from build123d import *

# Parameters (mm, degrees)
SKETCH1_R           = 1.778
SKETCH1_W           = 25.4
SKETCH1_H           = 5.842
BOSS_EXTRUDE1_DEPTH = 5.842
SKETCH2_W           = 63.5
SKETCH2_H           = 6.757924
BOSS_EXTRUDE2_DEPTH = 5.842
FILLET1_R           = 3.175
SKETCH4_R           = 3.175
SKETCH4_W           = 2.975
SKETCH4_H           = 6.35
CUT_EXTRUDE2_DEPTH  = 95.65387769
CUT_EXTRUDE3_DEPTH  = 95.65387769
BOSS_EXTRUDE4_START = -5.842
SKETCH7_R           = 2.0828
BOSS_EXTRUDE4_DEPTH = 5.842
FILLET12_R          = 12.7
SKETCH8_R           = 2.0828
BOSS_EXTRUDE5_DEPTH = 5.842
FILLET13_R          = 3.175
SKETCH9_R           = 2.0828
CUT_EXTRUDE4_DEPTH  = 107.047047485


with BuildPart() as part:
    # Sketch1 → Boss-Extrude1 (new body)
    with BuildSketch(Plane.XY):
        Polygon((0, 12.7), (-5.842, 12.7), (-5.842, 0), (0, 0), (0, -12.7), (-5.842, -12.7), (-5.842, -25.4), (0, -25.4), (0, -25.908), (12.7, -25.908), (12.7, -31.75), (0, -31.75), (0, -38.1), (-5.842, -38.1), (-5.842, -50.8), (0, -50.8), (0, -57.349898), (12.7, -57.349898), (12.7, -63.191898), (25.4, -63.191898), (25.4, -57.349898), (50.8, -57.349898), (50.8, -63.191898), (63.5, -63.191898), (63.5, 17.55013), (0, 17.55013), align=None)
        with Locations((19.065986419, -60.397898)):
            Circle(SKETCH1_R, mode=Mode.SUBTRACT)
        with Locations((19.05, -28.702)):
            Circle(SKETCH1_R, mode=Mode.SUBTRACT)
        with Locations((57.157993209, -60.397898)):
            Circle(SKETCH1_R, mode=Mode.SUBTRACT)
        with Locations((38.1, -28.829)):
            Rectangle(SKETCH1_W, SKETCH1_H, mode=Mode.SUBTRACT)
        with Locations((57.15, -28.702)):
            Circle(SKETCH1_R, mode=Mode.SUBTRACT)
    extrude(amount=BOSS_EXTRUDE1_DEPTH)

    # Sketch2 → Boss-Extrude2 (add)
    with BuildSketch(Plane.XY.offset(5.842)):
        with Locations((31.75, -66.57086)):
            Rectangle(SKETCH2_W, SKETCH2_H)
    extrude(amount=-BOSS_EXTRUDE2_DEPTH)

    # Fillet1
    fillet1_edges = [part.edges().sort_by_distance(p)[0] for p in [
        (63.5, -69.949822, 2.921),
    ]]
    fillet(fillet1_edges, radius=FILLET1_R)

    # Sketch4 → Cut-Extrude2 (cut, through all)
    with BuildSketch(Plane.XY.offset(5.842)):
        with Locations((38.1, 9.61263)):
            Circle(SKETCH4_R)
        with Locations((23.9125, -6.35)):
            Rectangle(SKETCH4_W, SKETCH4_H)
        with Locations((23.9125, -19.05)):
            Rectangle(SKETCH4_W, SKETCH4_H)
        with Locations((52.2875, -19.05)):
            Rectangle(SKETCH4_W, SKETCH4_H)
        with Locations((52.2875, -6.35)):
            Rectangle(SKETCH4_W, SKETCH4_H)
    extrude(amount=-CUT_EXTRUDE2_DEPTH, mode=Mode.SUBTRACT)

    # Sketch5 → Cut-Extrude3 (cut, through all)
    with BuildSketch(Plane.XY.offset(5.842)):
        with BuildLine():
            Line((7.9375, 8.02513), (17.4625, 8.02513))
            ThreePointArc((17.4625, 8.02513), (20.6375, 4.85013), (17.4625, 1.67513))
            Line((17.4625, 1.67513), (7.9375, 1.67513))
            ThreePointArc((7.9375, 1.67513), (4.7625, 4.85013), (7.9375, 8.02513))
        make_face()
        with BuildLine():
            Line((7.9375, -1.62687), (17.4625, -1.62687))
            ThreePointArc((17.4625, -1.62687), (20.6375, -4.80187), (17.4625, -7.97687))
            Line((17.4625, -7.97687), (7.9375, -7.97687))
            ThreePointArc((7.9375, -7.97687), (4.7625, -4.80187), (7.9375, -1.62687))
        make_face()
        with BuildLine():
            Line((7.9375, -11.27887), (17.4625, -11.27887))
            ThreePointArc((17.4625, -11.27887), (20.6375, -14.45387), (17.4625, -17.62887))
            Line((17.4625, -17.62887), (7.9375, -17.62887))
            ThreePointArc((7.9375, -17.62887), (4.7625, -14.45387), (7.9375, -11.27887))
        make_face()
    extrude(amount=-CUT_EXTRUDE3_DEPTH, mode=Mode.SUBTRACT)

    # Sketch7 → Boss-Extrude4 (add)
    with BuildSketch(Plane.XY.offset(5.842).offset(BOSS_EXTRUDE4_START)):
        with BuildLine():
            Line((60.544173966, -77.950003252), (55.218486469, -69.949822))
            Line((55.218486469, -69.949822), (60.325, -69.949822))
            ThreePointArc((60.325, -69.949822), (62.57006403, -69.01988603), (63.5, -66.774822))
            Line((63.5, -66.774822), (67.615323654, -70.182525218))
            ThreePointArc((67.615323654, -70.182525218), (68.150012892, -77.771642798), (60.544173966, -77.950003252))
        make_face()
        with Locations((64.262, -74.232177218)):
            Circle(SKETCH7_R, mode=Mode.SUBTRACT)
    extrude(amount=BOSS_EXTRUDE4_DEPTH)

    # Fillet12
    fillet12_edges = [part.edges().sort_by_distance(p)[0] for p in [
        (55.218486469, -69.949822, 2.921),
        (63.5, -66.774822, 2.921),
    ]]
    fillet(fillet12_edges, radius=FILLET12_R)

    # Sketch8 → Boss-Extrude5 (add)
    with BuildSketch(Plane.XY.offset(5.842)):
        with BuildLine():
            Line((64.693546, -17.610328), (63.5, -17.610328))
            Line((63.5, -17.610328), (63.5, -17.473065939))
            ThreePointArc((63.5, -17.473065939), (59.435746, -12.352528), (63.5, -7.231990061))
            Line((63.5, -7.231990061), (63.5, -7.094728))
            Line((63.5, -7.094728), (64.693546, -7.094728))
            ThreePointArc((64.693546, -7.094728), (69.951346, -12.352528), (64.693546, -17.610328))
        make_face()
        with Locations((64.693546, -12.352528)):
            Circle(SKETCH8_R, mode=Mode.SUBTRACT)
    extrude(amount=-BOSS_EXTRUDE5_DEPTH)

    # Fillet13
    # the kernel refuses this fillet: 3.175 mm, written as the material it adds along each edge
    with BuildSketch(Plane(origin=(63.5, -7.094728, 5.842), x_dir=(0, 1, 0), z_dir=(0, 0, -1))) as fillet13_piece_1:
        with BuildLine():
            CenterArc((2.938903965, 3.175), FILLET13_R, 193.589847282, 76.410152718)
            Line((-0.147204456, 2.428970633), (-0.455815298, 2.354367696))
            ThreePointArc((-0.455815298, 2.354367696), (-0.3175, 1.193546), (-0.3175, 0))
            Line((-0.3175, 0), (0, -0.3175))
            Line((0, -0.3175), (2.938903965, -0.3175))
            Line((2.938903965, -0.3175), (2.938903965, 0))
        make_face()
    extrude(amount=5.842)
    with BuildSketch(Plane(origin=(63.5, -17.610328, 5.842), x_dir=(0.9981686426778995, 0.0604926505830248, 0), z_dir=(0, 0, -1))) as fillet13_piece_2:
        with BuildLine():
            CenterArc((2.99140335, 3.125585947), FILLET13_R, 183.468090933, 76.410152718)
            Line((-0.177782091, 2.933521781), (-0.494700635, 2.914315365))
            Line((-0.494700635, 2.914315365), (-0.316918544, -0.019206417))
            Line((-0.316918544, -0.019206417), (0.019206417, -0.316918544))
            ThreePointArc((0.019206417, -0.316918544), (1.210566607, -0.244717783), (2.377629483, -0.312558595))
            Line((2.377629483, -0.312558595), (2.433427107, 0))
        make_face()
    extrude(amount=5.842)
    # the kernel refuses this fillet: 3.175 mm, written as the material it takes off along each edge

    # Sketch9 → Cut-Extrude4 (cut, through all)
    with BuildSketch(Plane.XY.offset(5.842)):
        with Locations((64.693546, -12.352528)):
            Circle(SKETCH9_R)
    extrude(amount=-CUT_EXTRUDE4_DEPTH, mode=Mode.SUBTRACT)


solid = part.part
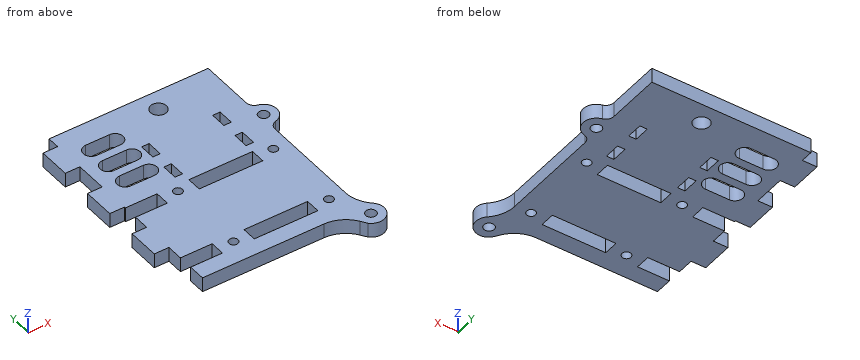
Geometry: final body of the model. Coordinates: model frame, mm. Round coordinates to 2 decimals unless told otherwise and drop trailing zeros. Loops run counter-clockwise (first coordinate to the right, second up) from the corner with the lowest first, then second, coordinate; pieces in that order, holes last.
Q1. Material intervals for L1, parallel to Y at x = 2.5, z = 4.9; L2, parallel to Y at x = 22.5, z = 0.3 (3 decimals); L3, parallel to Y at x = 20, z = 3.55, sorted ascending.
Q2. Section D-D on y = -46. Return loops of the section in (x, z), plus the area to 3 significant figures.
Q3. Section A-A on x = 32.5. Return loops of the section in (y, z).
Q4. Pin query (flat end, axial travel): P1, Ø1, axis at x = 36, z = 1.5, coming from the -Y side; P2, Ø2.5, axis at x = 52, z = 4, coming from the -Y side; P3, Ø1.8, axis at x = -2, z = 2, coming from the +Y side. Return the tip coordinate at first contact, or that it passes through.
Q5. Section B-B on x = 19.05. Return loops of the section in (y, z).
Q6. Section C-C on x = 57.15. Return loops of the section in (y, z).
Evaluation:
1. L1: y = -69.95 to -63.19, -57.35 to -31.75, -25.91 to 17.55
1. L2: y = -69.95 to -22.225, -15.875 to -9.525, -3.175 to 17.55
1. L3: y = -69.95 to -61.91, -58.88 to -30.2, -27.2 to -16.36, -12.55 to -6.71, -2.89 to 2.94, 6.76 to 17.55
2. outline: (-5.84, 0) - (63.5, 0) - (63.5, 5.84) - (-5.84, 5.84) - close
2. area: 405 mm2
3. outline: (-69.95, 0) - (-63.19, 0) - (-63.19, 5.84) - (-69.95, 5.84) - close; (-57.35, 0) - (-31.75, 0) - (-31.75, 5.84) - (-57.35, 5.84) - close; (-25.91, 0) - (17.55, 0) - (17.55, 5.84) - (-25.91, 5.84) - close
4. P1: stops at y = -69.95
4. P2: stops at y = -70.91
4. P3: stops at y = 12.7
5. outline: (-69.95, 0) - (-62.18, 0) - (-62.18, 5.84) - (-69.95, 5.84) - close; (-58.62, 0) - (-30.48, 0) - (-30.48, 5.84) - (-58.62, 5.84) - close; (-26.92, 0) - (-17.2, 0) - (-17.2, 5.84) - (-26.92, 5.84) - close; (-11.7, 0) - (-7.55, 0) - (-7.55, 5.84) - (-11.7, 5.84) - close; (-2.05, 0) - (2.1, 0) - (2.1, 5.84) - (-2.05, 5.84) - close; (7.6, 0) - (17.55, 0) - (17.55, 5.84) - (7.6, 5.84) - close
6. outline: (-73.43, 0) - (-62.18, 0) - (-62.18, 5.84) - (-73.43, 5.84) - close; (-58.62, 0) - (-30.48, 0) - (-30.48, 5.84) - (-58.62, 5.84) - close; (-26.92, 0) - (17.55, 0) - (17.55, 5.84) - (-26.92, 5.84) - close
